from build123d import *

# Parameters (mm, degrees)
SKETCH1_W           = 11.84764794
SKETCH1_H           = 16.748729175
BOSS_EXTRUDE1_DEPTH = 11
SKETCH1_3_R         = 0.6999986
SKETCH1_3_W         = 1.3999972
SKETCH1_3_H         = 1.3999972
SKETCH1_3_R_2       = 1.1500104
BOSS_EXTRUDE2_DEPTH = 4


with BuildPart() as part:
    # Sketch1 → Boss-Extrude1 (new body)
    with BuildSketch(Plane.XY):
        with Locations((0, -2.040885412)):
            Rectangle(SKETCH1_W, SKETCH1_H)
    extrude(amount=-BOSS_EXTRUDE1_DEPTH)

    # Sketch1_3 → Boss-Extrude2 (add)
    with BuildSketch(Plane.XY):
        with BuildLine():
            ThreePointArc((5.92382397, 1.1500104), (4.77381357, 0), (5.92382397, -1.1500104))
            Line((5.92382397, -1.1500104), (5.92382397, 1.1500104))
        make_face()
        with BuildLine():
            Line((5.92382397, 1.1500104), (5.92382397, -1.1500104))
            ThreePointArc((5.92382397, -1.1500104), (6.737004122, -0.813180152), (7.07383437, 0))
            ThreePointArc((7.07383437, 0), (6.737004122, 0.813180152), (5.92382397, 1.1500104))
        make_face()
        with Locations((-1.27, 2.117515676)):
            Circle(SKETCH1_3_R)
        with Locations((1.27, 4.657515676)):
            Circle(SKETCH1_3_R)
        with Locations((-1.27, 4.657515676)):
            Rectangle(SKETCH1_3_W, SKETCH1_3_H)
        with Locations(Location((-5.92382397, 0, 0), (0, 0, 270))):
            Circle(SKETCH1_3_R_2)
        with Locations((1.27, 2.117515676)):
            Circle(SKETCH1_3_R)
    extrude(amount=BOSS_EXTRUDE2_DEPTH)


solid = part.part
Can you work these out from the model? Positions are in its coordinate system, mm. A direction names the side the tool comes from. Coordinates: 2 decimals unless noted, no trailing zeros. Write each loop counter-clockwise with the first axis right and the second up, starting at its lowest first coordinate (ties: lowest second). Pieces come first, ordered by that corner, then holes. Notation, with made-up numbers: (19, 35.5) -> (39, 35.5) arc R25 cw to (39, 70.5) -> close; hole circle Ø3 at (34.25, 64). An arc over 180 degrees is marked (long way). Write item = value, one per line.
(1) If I drill on probe 1 along X at (y, z) = (-2.25, -3.5); probe 2 along Z at (x, y) = (0.75, -3); probe 3 along Y at (x, z) = (-1.75, 0.75), over which ranges is the centre line in solid material (lowest first)?
Verdict:
probe_1 = -5.92 to 5.92
probe_2 = -11 to 0
probe_3 = 1.61 to 2.63, 3.96 to 5.36
(2) On a 3-axis mill with a long thin cutter (end or side, diameter ignored), from which of +Z, -Z, +X, -X, +Y, -Y can I reach the whole of each face in a straight line? I mean faces 1 (the face through (-1.97, 5, 2)), 2 (the face through (0, -2, 0)), 3 (the face through (6.4, 0, 0)), 4 (the face through (-0.57, 5, 2)). Say none if no direction works.
Verdict:
face_1 = +Z, -X, +Y, -Y
face_2 = +Z
face_3 = -Z, +X, +Y, -Y
face_4 = +Z, +Y, -Y
(3) Imagine slicing it at A-A (x = -1.27). Please give me the cut outline in (y, z).
Verdict:
outline = (-10.42, -11) -> (6.33, -11) -> (6.33, 0) -> (5.36, 0) -> (5.36, 4) -> (3.96, 4) -> (3.96, 0) -> (2.82, 0) -> (2.82, 4) -> (1.42, 4) -> (1.42, 0) -> (-10.42, 0) -> close
(4) Imagine slicing it at D-D (z = -1). Please give me the cut outline in (x, y).
Verdict:
outline = (-5.92, -10.42) -> (5.92, -10.42) -> (5.92, 6.33) -> (-5.92, 6.33) -> close
(5) Imagine slicing it at C-C (y = -3.5). Please give me the cut outline in (x, z).
Verdict:
outline = (-5.92, -11) -> (5.92, -11) -> (5.92, 0) -> (-5.92, 0) -> close
(6) Thinking about a two-plate mould opening in Y: for faces 5 (the face through (-1, 5.358, 2)), 6 (the face through (0, -10.415, -5)), 7 (the face through (1.646, 2.708, 1.972)), which applies, +Y half, -Y half, draft (parallel to the pull), parting line (faces both ways), or undercut?
Verdict:
face_5 = +Y half
face_6 = -Y half
face_7 = undercut
(7) For pin 1 (1.3 mm diameter, centred on x = -6.5, y = 0.5, fed in from -Z); pin 2 (6 mm diameter, centred on y = 2.5, z = -2, fed in from +X); pin 3 (1.5 mm diameter, centred on y = 4.5, z = 1, fed in from -X); pin 4 (8 mm diameter, centred on x = -1, y = -5, fed in from +Z), each with a flat end and sliding along its axis, tell me the tip position at first contact or that it passes through.
Verdict:
pin_1 = -11
pin_2 = 7.04
pin_3 = -1.97
pin_4 = 0
(8) Imagine slicing it at B-B (z = 0.5). Please give me the cut outline in (x, y), and give its area (3 significant figures).
Verdict:
outline = circle Ø2.3 at (-5.92, 0); circle Ø1.4 at (-1.27, 2.12); (-1.97, 3.96) -> (-0.57, 3.96) -> (-0.57, 5.36) -> (-1.97, 5.36) -> close; circle Ø1.4 at (1.27, 2.12); circle Ø1.4 at (1.27, 4.66); circle Ø2.3 at (5.92, 0)
area = 14.9 mm^2
